For this review, take the finished solid that the model builds, in its own axes (mm). A direction names the side the tool comes from. Round coordinates to 2 decimals unless told otherwise and drop trailing zeros. Loops run counter-clockwise (first coordinate to the right, second up) from the corner with the lowest first, then second, coordinate; pieces in that order, holes last. Notation, with made-up numbers: (28.5, 74) -> (78.5, 74) arc R23 ccw to (78.5, 100) -> close; hole circle Ø11 at (8, 8). An arc over 180 degrees is marked (long way). Write each question's results on one line, items separated by ' | '.
Autodesk Inventor part; units mm, degrees
ref_plane "YZ Plane" through (0, 0, 0) normal (1, 0, 0) x (0, 1, 0)
ref_plane "XZ Plane" through (0, 0, 0) normal (0, 1, 0) x (-1, 0, 0)
ref_plane "XY Plane" through (0, 0, 0) normal (0, 0, 1) x (1, 0, 0)
sketch "スケッチ1" plane through (0, 0, 0) normal (0, 0, 1) x (1, 0, 0)
  line L0 (-60, 100) -> (60, 100)
  line L1 (60, 100) -> (60, -100)
  line L2 (60, -100) -> (-60, -100)
  line L3 (-60, -100) -> (-60, 100)
  line L4 (60, 117.6777) -> (77.6777, 100)
  line L5 (77.6777, 100) -> (60, 82.3223)
  line L6 (60, 82.3223) -> (42.3223, 100)
  line L7 (42.3223, 100) -> (60, 117.6777)
  line L8 (60, -82.3223) -> (77.6777, -100)
  line L9 (77.6777, -100) -> (60, -117.6777)
  line L10 (60, -117.6777) -> (42.3223, -100)
  line L11 (42.3223, -100) -> (60, -82.3223)
  line L12 (-60, -82.3223) -> (-42.3223, -100)
  line L13 (-42.3223, -100) -> (-60, -117.6777)
  line L14 (-60, -117.6777) -> (-77.6777, -100)
  line L15 (-77.6777, -100) -> (-60, -82.3223)
  line L16 (-60, 117.6777) -> (-42.3223, 100)
  line L17 (-42.3223, 100) -> (-60, 82.3223)
  line L18 (-60, 82.3223) -> (-77.6777, 100)
  line L19 (-77.6777, 100) -> (-60, 117.6777)
  point P0 (0, 0)
  dimension "d0" = 200
  dimension "d1" = 100
  dimension "d2" = 120
  dimension "d3" = 60
  dimension "d4" = 12.5
  dimension "d5" = 12.5
  dimension "d6" = 12.5
  dimension "d7" = 12.5
extrude "押し出し1" add sketch "スケッチ1" along normal blind 2
sketch "スケッチ2" plane through (0, 0, 2) normal (0, 0, 1) x (1, 0, 0)
  line L0 (77.6777, 100) -> (60, 82.3223)
  line L1 (60, 117.6777) -> (77.6777, 100)
  line L2 (42.3223, 100) -> (60, 117.6777)
  line L3 (-60, 117.6777) -> (-42.3223, 100)
  line L4 (-77.6777, 100) -> (-60, 117.6777)
  line L5 (-60, 82.3223) -> (-77.6777, 100)
  line L6 (-77.6777, -100) -> (-60, -82.3223)
  line L7 (-60, -117.6777) -> (-77.6777, -100)
  line L8 (-42.3223, -100) -> (-60, -117.6777)
  line L9 (60, -117.6777) -> (42.3223, -100)
  line L10 (77.6777, -100) -> (60, -117.6777)
  line L11 (60, -82.3223) -> (77.6777, -100)
  circle A0 centre (-46.2114, -74.8977) radius 1.5
  circle A1 centre (-34.8977, -86.2114) radius 1.5
  circle A2 centre (34.8977, -86.2114) radius 1.5
  circle A3 centre (46.2114, -74.8977) radius 1.5
  circle A4 centre (46.2114, 74.8977) radius 1.5
  circle A5 centre (34.8977, 86.2114) radius 1.5
  circle A6 centre (-34.8977, 86.2114) radius 1.5
  circle A7 centre (-46.2114, 74.8977) radius 1.5
  point P0 (0, 0)
  dimension "d10" = 3
  dimension "d12" = 40
  dimension "d13" = 40
  dimension "d14" = 4.5
  dimension "d15" = 4.5
  dimension "d16" = 40
  dimension "d17" = 40
  dimension "d18" = 40
  dimension "d19" = 40
  dimension "d20" = 40
  dimension "d21" = 40
  dimension "d22" = 4.5
  dimension "d23" = 4.5
  dimension "d24" = 4.5
  dimension "d25" = 4.5
  dimension "d26" = 4.5
  dimension "d27" = 4.5
hole "穴1" at (34.8977, -86.2114, 2) at (46.2114, -74.8977, 2) at (-34.8977, -86.2114, 2) at (-46.2114, -74.8977, 2) at (34.8977, 86.2114, 2) at (46.2114, 74.8977, 2) at (-46.2114, 74.8977, 2) at (-34.8977, 86.2114, 2) direction (0, 0, -1) diameter 3 end through all
sketch "スケッチ3" plane through (0, 0, 2) normal (0, 0, 1) x (1, 0, 0)
  line L0 (77.6777, 100) -> (60, 82.3223)
  line L1 (60, 117.6777) -> (77.6777, 100)
  line L2 (42.3223, 100) -> (60, 117.6777)
  line L3 (-60, 117.6777) -> (-42.3223, 100)
  line L4 (-77.6777, 100) -> (-60, 117.6777)
  line L5 (-60, 82.3223) -> (-77.6777, 100)
  line L6 (-77.6777, -100) -> (-60, -82.3223)
  line L7 (-60, -117.6777) -> (-77.6777, -100)
  line L8 (-42.3223, -100) -> (-60, -117.6777)
  line L9 (60, -117.6777) -> (42.3223, -100)
  line L10 (77.6777, -100) -> (60, -117.6777)
  line L11 (60, -82.3223) -> (77.6777, -100)
  circle A0 centre (-39.1403, 90.4541) radius 2.25
  circle A1 centre (-50.4541, 79.1403) radius 2.25
  circle A2 centre (-50.4541, -79.1403) radius 2.25
  circle A3 centre (-39.1403, -90.4541) radius 2.25
  circle A4 centre (39.1403, -90.4541) radius 2.25
  circle A5 centre (50.4541, -79.1403) radius 2.25
  circle A6 centre (50.4541, 79.1403) radius 2.25
  circle A7 centre (39.1403, 90.4541) radius 2.25
  point P0 (0, 0)
  dimension "d35" = 4.5
  dimension "d37" = 4.5
  dimension "d38" = 4.5
  dimension "d39" = 34
  dimension "d40" = 34
  dimension "d41" = 4.5
  dimension "d42" = 4.5
  dimension "d43" = 34
  dimension "d44" = 34
  dimension "d45" = 34
  dimension "d46" = 4.5
  dimension "d47" = 4.5
  dimension "d48" = 34
  dimension "d49" = 34
  dimension "d50" = 34
  dimension "d51" = 4.5
  dimension "d52" = 4.5
hole "穴2" at (-50.4541, -79.1403, 2) at (-39.1403, -90.4541, 2) at (39.1403, 90.4541, 2) at (50.4541, 79.1403, 2) at (-50.4541, 79.1403, 2) at (-39.1403, 90.4541, 2) at (39.1403, -90.4541, 2) at (50.4541, -79.1403, 2) direction (0, 0, -1) diameter 4.5 end through all
sketch "スケッチ4" plane through (0, 0, 2) normal (0, 0, 1) x (1, 0, 0)
  line L0 (77.6777, 100) -> (60, 82.3223)
  line L1 (60, 117.6777) -> (77.6777, 100)
  line L2 (42.3223, 100) -> (60, 117.6777)
  line L3 (-60, 117.6777) -> (-42.3223, 100)
  line L4 (-77.6777, 100) -> (-60, 117.6777)
  line L5 (-60, 82.3223) -> (-77.6777, 100)
  line L6 (-77.6777, -100) -> (-60, -82.3223)
  line L7 (-60, -117.6777) -> (-77.6777, -100)
  line L8 (-42.3223, -100) -> (-60, -117.6777)
  line L9 (60, -117.6777) -> (42.3223, -100)
  line L10 (77.6777, -100) -> (60, -117.6777)
  line L11 (60, -82.3223) -> (77.6777, -100)
  line L12 (-60, -82.3223) -> (-42.3223, -100)
  line L13 (42.3223, -100) -> (60, -82.3223)
  line L14 (42.3223, 100) -> (60, 82.3223)
  line L15 (-60, 82.3223) -> (-42.3223, 100)
  point P0 (0, 0)
  dimension "d60" = 25
  dimension "d61" = 25
  dimension "d62" = 25
  dimension "d63" = 25
extrude "押し出し2" cut sketch "スケッチ4" against normal blind 3
sketch "スケッチ6" plane through (-42.3223, 100, 0) normal (0, 1, 0) x (1, 0, 0)
  line L0 (84.6447, 0) -> (0, 0)
  line L1 (0, -2) -> (84.6447, -2)
  line L2 (29.8223, 0) -> (54.8223, 0)
  line L3 (54.8223, 0) -> (54.8223, -2)
  line L4 (54.8223, -2) -> (29.8223, -2)
  line L5 (29.8223, -2) -> (29.8223, 0)
  point P0 (42.3223, 0)
  dimension "d66" = 25
  dimension "d68" = 12.5
extrude "押し出し3" add sketch "スケッチ6" along normal blind 10
sketch "スケッチ7" plane through (0, 0, 2) normal (0, 0, 1) x (1, 0, 0)
  line L0 (-12.5, 110) -> (12.5, 110)
  line L1 (-12.5, 100) -> (-12.5, 110)
  circle A0 centre (-8, 98) radius 1.5
  circle A1 centre (8, 98) radius 1.5
  point P0 (0, 0)
  dimension "d71" = 16
  dimension "d72" = 12
  dimension "d73" = 12
  dimension "d74" = 3
  dimension "d75" = 4.5
hole "穴3" at (-8, 98, 2) at (8, 98, 2) direction (0, 0, -1) diameter 3 end through all
sketch "スケッチ10" plane through (0, 0, 2) normal (0, 0, 1) x (1, 0, 0)
  line L0 (42.3223, -100) -> (-42.3223, -100)
  line L1 (-60, -82.3223) -> (-60, 82.3223)
  arc A0 (6.5, 27) -> (-6.5, 27) centre (0, 27) ccw
  arc A1 (-6.5, 0) -> (6.5, 0) centre (0, 0) ccw
  line L2 (-6.5, 27) -> (-6.5, 0)
  line L3 (6.5, 27) -> (6.5, 0)
  point P0 (0, 0)
  dimension "d116" = 13
  dimension "d118" = 27
  dimension "d119" = 60
  dimension "d120" = 100
  dimension "d121" = 60
  dimension "d122" = 27
extrude "押し出し4" cut sketch "スケッチ10" against normal blind 2
sketch "スケッチ11" plane through (0, 0, 2) normal (0, 0, 1) x (1, 0, 0)
  arc A0 (6.5, 27) -> (-6.5, 27) centre (0, 27) ccw
  circle A1 centre (-8, 31.5) radius 1
  circle A2 centre (-8, -4.5) radius 1
  circle A3 centre (8, -4.5) radius 1
  circle A4 centre (8, 31.5) radius 1
  point P0 (0, 0)
  dimension "d125" = 2
  dimension "d127" = 16
  dimension "d128" = 8
  dimension "d129" = 16
  dimension "d130" = 8
  dimension "d131" = 36
  dimension "d132" = 36
  dimension "d133" = 4.5
  dimension "d134" = 4.5
hole "穴6" at (-8, 31.5, 2) at (-8, -4.5, 2) at (8, -4.5, 2) at (8, 31.5, 2) direction (0, 0, -1) diameter 2 depth 2 tip angle 118 counterbore diameter 4 counterbore depth 0.5
equation "\"d33\" = d26"
equation "\"d58\" = d46"
properties material "アルミニウム 6061"
1. Consider section B-B (y = 22.5). State the section outline as (x, z) points, plus the area to 3 significant figures.
Values found:
outline: (-60, 0) -> (-6.5, 0) -> (-6.5, 2) -> (-60, 2) -> close; (6.5, 0) -> (60, 0) -> (60, 2) -> (6.5, 2) -> close | area: 214 mm2
2. Tool access review of faces 5 (the face through (-0.1, -6.5, 1)), 6 (the face through (-14, 6, 0)), 7 (the face through (-7.1, -5.4, 1.5)): name each direction out of +Z, -Z, +X, -X, +Y, -Y from which nothing blocks a thin tool from reaching the whole face with its end or side.
Values found:
face 5: +Z, -Z | face 6: -Z, +X, -X, +Y, -Y | face 7: +Z
3. Consider section A-A (x = 0). State the section outline as (y, z) points, plus the area to 3 significant figures.
Values found:
outline: (-100, 0) -> (-6.5, 0) -> (-6.5, 2) -> (-100, 2) -> close; (33.5, 0) -> (110, 0) -> (110, 2) -> (33.5, 2) -> close | area: 340 mm2
4. Consider section C-C (z = 0.5). Give the number of separate pieces and of enclosed holes in the cut face, plus the area to 3 significant figures.
Values found:
separate pieces: 1 | enclosed holes: 23 | area: 22,900 mm2
5. To check wall thickness, follow probe 1 along Y at (x, z) = (8, 1.05); probe 2 along Y at (x, z) = (35, 1.8); probe 3 along X at (y, z) = (10, 0.2). State the ranges of each line that lie inside material, in increasing order.
Values found:
probe 1: y = -100 to -5.5, -3.5 to 30.5, 32.5 to 96.5, 99.5 to 110 | probe 2: y = -100 to -87.71, -84.71 to 84.71, 87.71 to 100 | probe 3: x = -60 to -6.5, 6.5 to 60
6. Draft analysis for pull direction Y (two halves, no side actions). For faces 1 (the face through (51.04, -91.28, 1.01)), 2 (the face through (-14, 6, 2)), 3 (the face through (-51.97, -77.48, 0.99)), 4 (the face through (-51.28, 91.04, 1.01)), state which applies: released by +Y, released by -Y, zero draft, split by the parting line, or undercut.
Values found:
face 1: released by -Y | face 2: zero draft | face 3: undercut | face 4: released by +Y
7. For pin 1 (2.5 mm diameter, centred on x = 8, y = -4.5, fed in from -Z); pin 2 (1.2 mm diameter, centred on x = 8.5, y = -4, fed in from +Z), all flat-tipped, find the tip position at first contact; note any pin that passes through.
Values found:
pin 1: stops at z = 0 | pin 2: stops at z = 1.5
8. Consider section D-D (x = 15.5). State the section outline as (y, z) points.
Values found:
outline: (-100, 0) -> (100, 0) -> (100, 2) -> (-100, 2) -> close
